Verification items for this drawing (mm, ordinates from the low corner). A direction names the side the tool comes from. Round coordinates to 2 decimals unless told otherwise and drop trailing zeros. Write each loop counter-clockwise with the first axis right and the second up, starting at its lowest first coordinate (ties: lowest second). Pieces come first, ordered by that corner, then holes.
Item 1: Cross-section at A-A (x = 12.7). Enter the section's corners in (y, z) (1 decimal).
Item 2: Cross-section at B-B (y = 6). Enter the section's corners in (x, z).
Item 3: Scan lines: probe 1 along Z at (x, y) = (10.5, 1.25); probe 2 along Y at (x, z) = (12.7, 4.75) (1 decimal); probe 3 along Y at (x, z) = (21.25, 5.5). Record each from-to range of solid material in increasing order.
Item 4: Access from +Z, -Z, +X, -X, +Y, -Y to the whole of each face (thin tool, end or side, straight path). Record for the marked faces 1, 2 and 3.
Item 5: Draft check along X on the marked faces 4, 5, 6 and 7. Enter one of: pulls with the +X half, pulls with the -X half, needs draft (parallel to the pull), parting line crosses it, or undercut.
Item 6: Depth check by flat-ended pin: P1, Ø1.9, axis at x = 13.5, z = 7, coming from the -Y side; P2, Ø1.2, axis at x = 18, y = 13.5, coming from the +Z side; P3, Ø4, axis at y = 14, z = 3.5, coming from the -X side; P4, Ø3, axis at x = 19, z = 6, coming from the +Y side. Enter the tip coordinate at first touch or a pass-through.
Item 7: Cross-section at D-D (x = 18). Enter the section's corners in (y, z) (1 decimal).
Item 8: Cross-section at C-C (z = 6.5). Enter the section's corners in (x, y) (1 decimal).
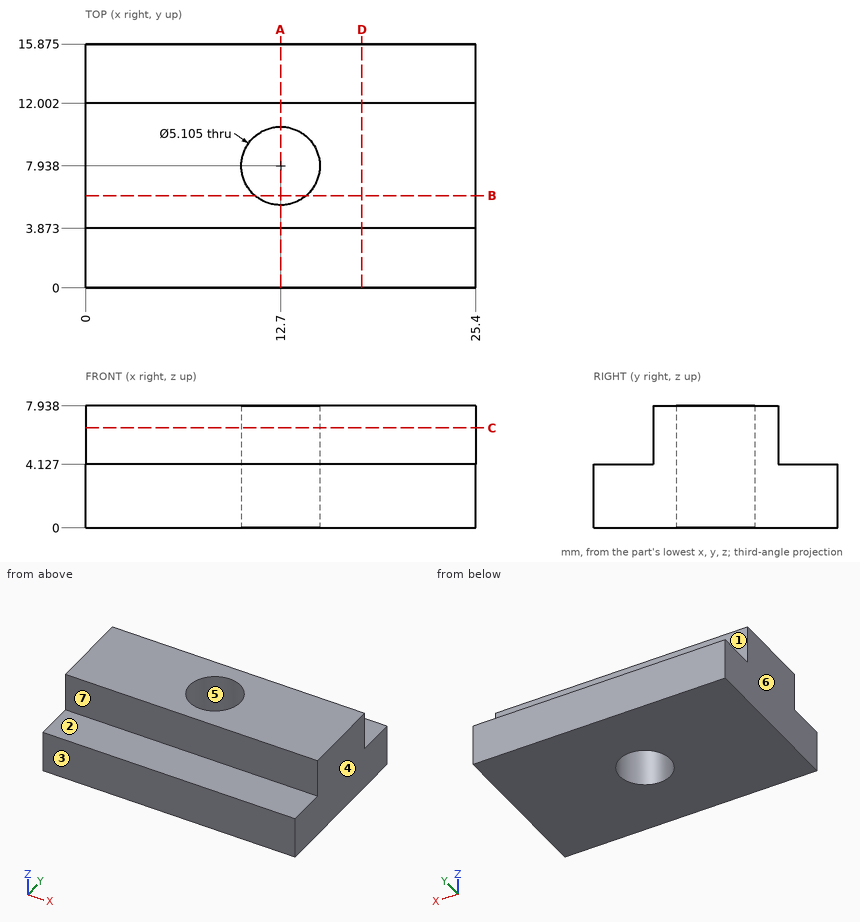
Resolved:
1. outline: (0, 0) - (5.4, 0) - (5.4, 7.9) - (3.9, 7.9) - (3.9, 4.1) - (0, 4.1) - close; (10.5, 0) - (15.9, 0) - (15.9, 4.1) - (12, 4.1) - (12, 7.9) - (10.5, 7.9) - close
2. outline: (0, 0) - (11.04, 0) - (11.04, 7.94) - (0, 7.94) - close; (14.36, 0) - (25.4, 0) - (25.4, 7.94) - (14.36, 7.94) - close
3. probe 1: z = 0 to 4.13
3. probe 2: y = 3.9 to 5.4, 10.5 to 12
3. probe 3: y = 3.87 to 12
4. face 1: +Z, +X, -X, +Y
4. face 2: +Z, +X, -X, -Y
4. face 3: +Z, -Z, +X, -X, -Y
5. face 4: pulls with the +X half
5. face 5: undercut
5. face 6: pulls with the -X half
5. face 7: needs draft
6. P1: stops at y = 3.87
6. P2: stops at z = 4.13
6. P3: stops at x = 0
6. P4: stops at y = 12
7. outline: (0, 0) - (15.9, 0) - (15.9, 4.1) - (12, 4.1) - (12, 7.9) - (3.9, 7.9) - (3.9, 4.1) - (0, 4.1) - close
8. outline: (0, 3.9) - (25.4, 3.9) - (25.4, 12) - (0, 12) - close; hole circle Ø5.1 at (12.7, 7.9)
